Here's the drawing with two shaded views (mm, measured from the low corner). I have some questions. A direction names the side the tool comes from. Round coordinates to 2 decimals unless told otherwise and drop trailing zeros. Loops run counter-clockwise (first coordinate to the right, second up) from the corner with the lowest first, then second, coordinate; pieces in that order, holes last.
(1) I want a section at A-A on y = 33. Write out the boundary of the cut face in (x, z), plus the area to 3 significant figures.
(2) Thinking about a two-plate mould opening in X: for the marked faces 1, 2, 3 and 4, which applies, released by +X, released by -X, zero draft, split by the parting line, or undercut?
(3) Will these pins go through, and if not, where does the flat tip stop? pin 1 Ø3.5 at (x, z) = (52, 6) entering from -Y; pin 2 Ø10 at (y, z) = (10.5, 13.5) entering from -X; pin 3 Ø8 at (x, z) = (13, 13) entering from +Y; pin 4 Ø3 at (x, z) = (2.51, 5) entering from +Y.
(4) I want a section at D-D on x = 37.25. Write out the boundary of the cut face in (y, z) (1 decimal).
(5) If I drill on line 1 along Z through (x, y) = (51, 32) (1 decimal); line 2 along Z through (x, y) = (2, 29); line 3 along Y through (x, z) = (6.5, 6.5), over which ranges is the centre line in solid material (lowest first)?
(6) Which directions (+Z, -Z, +X, -X, +Y, -Y) give clear straight access to the entire face, cutting with the end or side of a thin tool? Please do the marked faces 5, 6, 7, 8 and 9.
(7) I want a section at C-C on z = 15. Give the number of separate pieces and of enclosed holes in the cut face, plus the area to 3 significant figures.
(8) I want a section at B-B on x = 51.99. Write out the boundary of the cut face in (y, z).
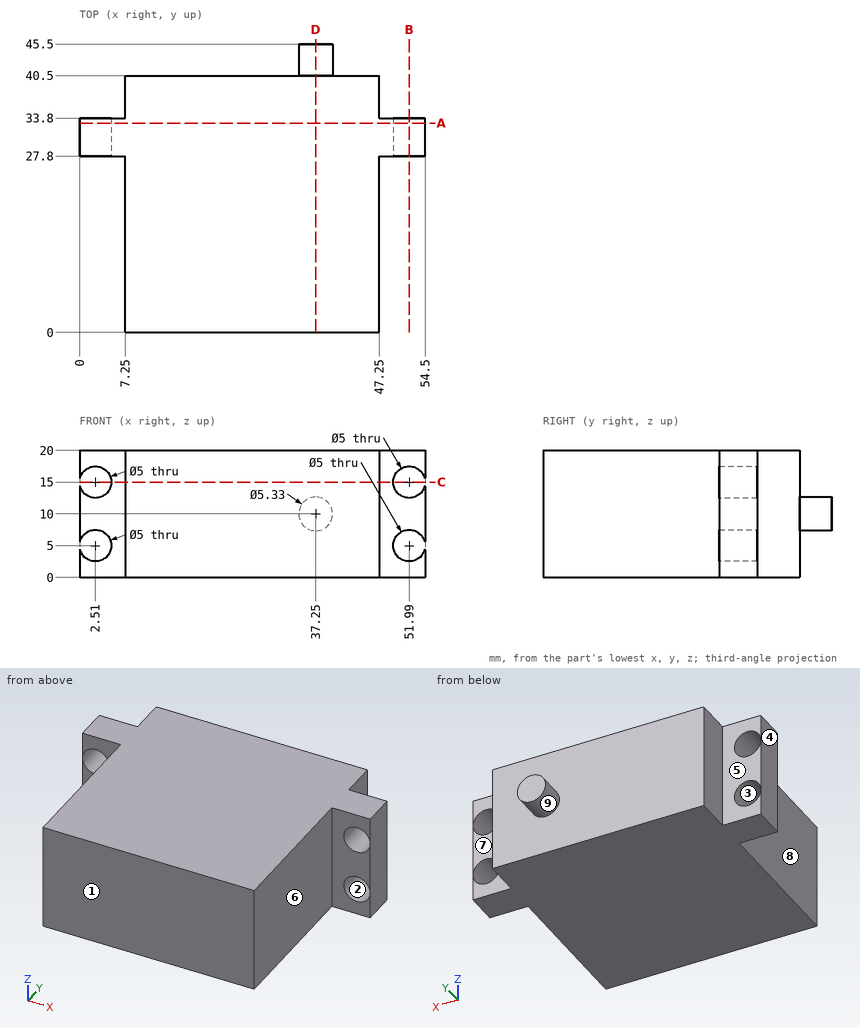
Filled sheet:
1. outline: (0, 0) - (54.5, 0) - (54.5, 20) - (0, 20) - close; hole circle Ø5 at (2.51, 5); hole circle Ø5 at (2.51, 15); hole circle Ø5 at (51.99, 5); hole circle Ø5 at (51.99, 15)
1. area: 1,010 mm2
2. face 1: zero draft
2. face 2: undercut
2. face 3: undercut
2. face 4: released by -X
3. pin 1: stops at y = 27.8
3. pin 2: stops at x = 7.25
3. pin 3: stops at y = 40.5
3. pin 4: passes through
4. outline: (0, 0) - (40.5, 0) - (40.5, 7.3) - (45.5, 7.3) - (45.5, 12.7) - (40.5, 12.7) - (40.5, 20) - (0, 20) - close
5. line 1: z = 0 to 2.7, 7.3 to 12.7, 17.3 to 20
5. line 2: z = 0 to 2.55, 7.45 to 12.55, 17.45 to 20
5. line 3: y = 27.8 to 33.8
6. face 5: +Z, -Z, -X, +Y
6. face 6: +Z, -Z, +X, -Y
6. face 7: +Z, -Z, +X, +Y
6. face 8: +Z, -Z, -X, -Y
6. face 9: +Y
7. separate pieces: 3
7. enclosed holes: 0
7. area: 1,650 mm2
8. outline: (27.8, 0) - (33.8, 0) - (33.8, 2.5) - (27.8, 2.5) - close; (27.8, 7.5) - (33.8, 7.5) - (33.8, 12.5) - (27.8, 12.5) - close; (27.8, 17.5) - (33.8, 17.5) - (33.8, 20) - (27.8, 20) - close
